Geometry check sheet. Reference: drawing and pictorial views, mm from the part's lowest x, y, z. A direction names the side the tool comes from. Give positions to 0.01 mm unless a question says otherwise; leave off trailing zeros. Write each loop counter-clockwise with the first axis right and the second up, starting at its lowest first coordinate (ties: lowest second). Pieces come first, ordered by that corner, then holes.
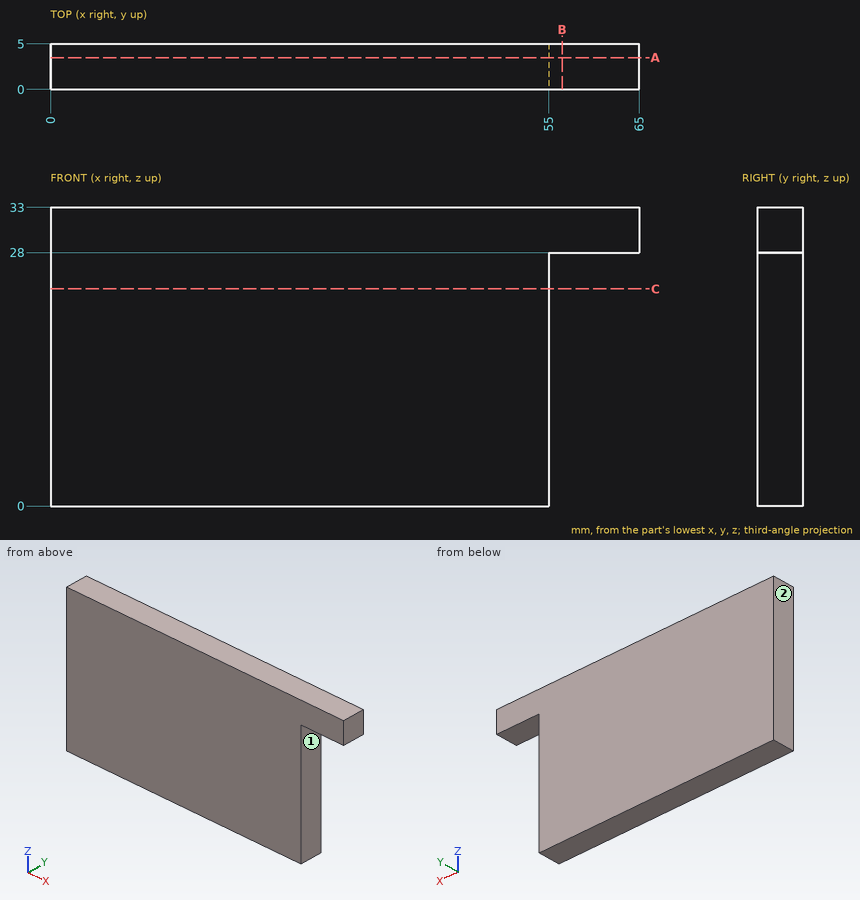
Item 1: Sectioned sample at B-B on x = 56.5. Record the cut outline in (y, z).
Answer key:
outline: (0, 28) - (5, 28) - (5, 33) - (0, 33) - close
Item 2: Depth check by flat-ended pin: pin 1 (4 mm diameter, centred on x = 55, z = 12, fed in from -Y); pin 2 (1 mm diameter, centred on y = 3, z = 15.5, fed in from +X). Enter the tip coordinate at first touch or a pass-through.
Answer key:
pin 1: stops at y = 0
pin 2: stops at x = 55
Item 3: Scan line: line 1 along X through (y, z) = (2.05, 27.5). Record every from-to range of solid material in increasing order.
Answer key:
line 1: x = 0 to 55
Item 4: Set-up check for the marked faces 1 and 2: record each of +Z, -Z, +X, -X, +Y, -Y from which the full face is reachable in a straight line by a thin tool's end or side.
Answer key:
face 1: -Z, +X, +Y, -Y
face 2: +Z, -Z, -X, +Y, -Y
Item 5: Sectioned sample at A-A on y = 3.5. Record the cut outline in (x, z).
Answer key:
outline: (0, 0) - (55, 0) - (55, 28) - (65, 28) - (65, 33) - (0, 33) - close
Item 6: Sectioned sample at C-C on z = 24. Record the cut outline in (x, y).
Answer key:
outline: (0, 0) - (55, 0) - (55, 5) - (0, 5) - close
